For this review, use the dimensioned drawing (mm, ordinates from the lowest corner) and the shaded views. A direction names the side the tool comes from. Give positions to 0.01 mm unless a question says otherwise; leave off trailing zeros. Order: outer loops, then holes, each group sorted by start corner. A loop starts at its lowest first (then second) coordinate and runs counter-clockwise, first axis right, second up. Notation, with made-up numbers: M -27,31.5 L 32,31.5 A11 ccw 32,52.5 Z; hole C -37,-36.5 d7. An arc over 180 degrees is marked long. One line per question, with ' | ' between items. Start each with the question number.
1. Insertion check: P1, Ø3, axis at x = 72.5, z = 13, coming from the -Y side; P2, Ø4.5, axis at x = 95.5, y = 2.5, coming from the +Z side; P3, Ø2.5, axis at x = 56.5, z = 18, coming from the -Y side; P4, Ø12, axis at x = 28, y = 30.5, coming from the -Z side. Each pin has a flat end and moves straight along its axis. Give the tip position at first contact, or say it passes through.
2. We need section A-A on x = 2.5. Write out the cut boundary in (y, z).
3. For the marked faces 1 and 2, list the 3-axis set-ups (+Z, -Z, +X, -X, +Y, -Y) from which the entire face can be reached by the end or side of a thin tool; tool diameter is ignored.
4. We need section C-C on z = 18.25. Write out the cut boundary in (x, y), then the cut area to 3 significant figures.
5. We need section B-B on y = 2.5. Write out the cut boundary in (x, z), then the cut area to 3 significant figures.
6. Wall thickness on L1, parallel to Y at x = 2.5, z = 15.45; L2, parallel to Y at x = 36.5, z = 17.75; L3, parallel to Z at x = 76, y = 4: over which ranges is each line inside the solid? List them lowest first.
7. We need section D-D on x = 39. Write out the cut boundary in (y, z).
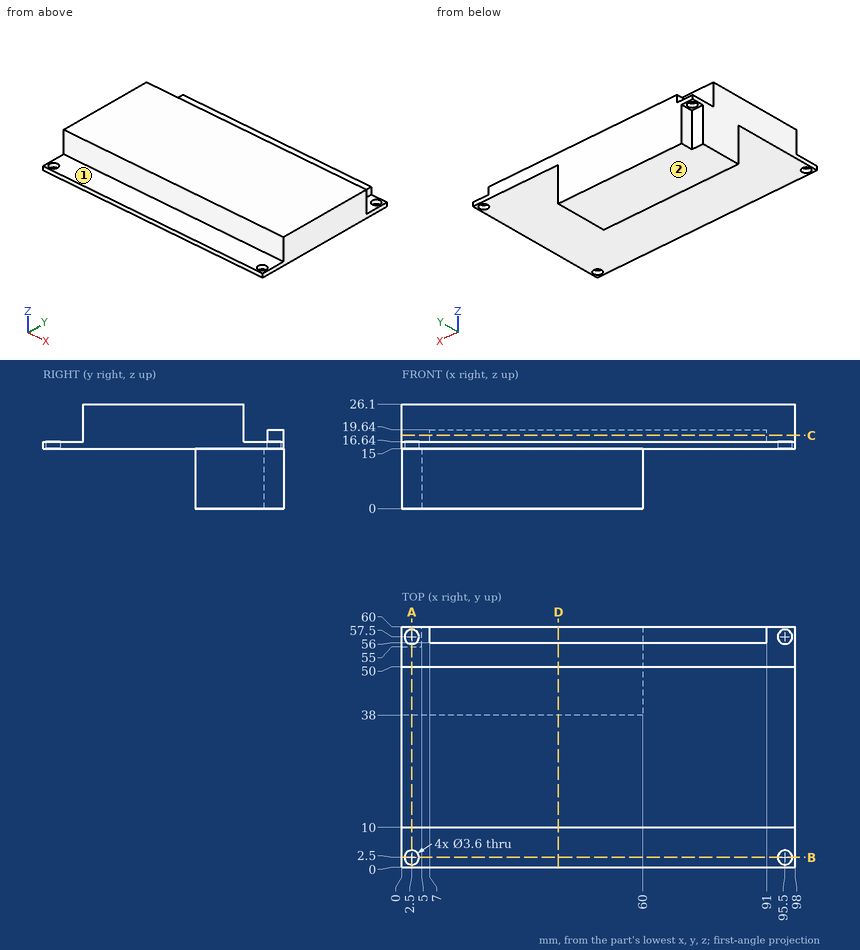
Entries:
1) P1: passes through | P2: stops at z = 16.64 | P3: stops at y = 10 | P4: stops at z = 15
2) outline: M 0,15 L 0.7,15 L 0.7,16.64 L 0,16.64 Z; M 4.3,15 L 38,15 L 38,0 L 55,0 L 55,15 L 55.7,15 L 55.7,16.64 L 50,16.64 L 50,26.1 L 10,26.1 L 10,16.64 L 4.3,16.64 Z; M 59.3,15 L 60,15 L 60,16.64 L 59.3,16.64 Z
3) face 1: +Z, +X, -X, -Y | face 2: -Z, +X, -X, +Y, -Y
4) outline: M 0,10 L 98,10 L 98,50 L 0,50 Z; M 7,56 L 91,56 L 91,60 L 7,60 Z | area: 4,260 mm^2
5) outline: M 0,15 L 0.7,15 L 0.7,16.64 L 0,16.64 Z; M 4.3,15 L 93.7,15 L 93.7,16.64 L 4.3,16.64 Z; M 97.3,15 L 98,15 L 98,16.64 L 97.3,16.64 Z | area: 149 mm^2
6) L1: y = 0 to 0.7, 4.3 to 55.7, 59.3 to 60 | L2: y = 10 to 50, 56 to 60 | L3: z = 15 to 16.64
7) outline: M 0,15 L 38,15 L 38,0 L 60,0 L 60,19.64 L 56,19.64 L 56,16.64 L 50,16.64 L 50,26.1 L 10,26.1 L 10,16.64 L 0,16.64 Z
